from build123d import *

# Parameters (mm, degrees)
F2_R           = 14.99999
F4_D           = 5
F4_CBORE_D     = 8
F4_CBORE_DEPTH = 2


# Not quite as in the source:
# - a fillet or chamfer is up to 0.001 mm smaller than in the source, because OpenCascade refuses the exact size


with BuildPart() as f1:
    # F0 (on Front) → F1 (revolve)
    with BuildSketch(Plane.XZ):
        Polygon((36, -25), (0, -25), (0, -30), (43.5, -30), (43.5, -15), (36, -15), align=None)
    revolve(axis=Axis((0, 0, -27.5), (0, 0, 1)))

    # F2 (radius 15 in the source; OpenCascade refuses exactly that, so slightly less here)
    f2_edges = [f1.edges().sort_by_distance(p)[0] for p in [
        (-43.5, 0, -30),
    ]]
    fillet(f2_edges, radius=F2_R)

    # F4 (through all)
    with Locations(Plane(origin=(0, 0, -30), x_dir=(1, 0, 0), z_dir=(0, 0, -1))):
        with Locations((-12.9903810568, 7.5), (12.9903810568, 7.5), (0, -15)):
            CounterBoreHole(F4_D / 2, F4_CBORE_D / 2, F4_CBORE_DEPTH)


solid = f1.part
Geometry: final body of the model. Coordinates: model frame, mm. A direction names the side the tool comes from. Coordinates: 2 decimals unless noted, no trailing zeros. Write each loop counter-clockwise with the first axis right and the second up, starting at its lowest first coordinate (ties: lowest second). Pieces come first, ordered by that corner, then holes. Notation, with made-up numbers: (-39.5, -23) - (6.5, -23) arc R20 ccw to (6.5, -10) - close; hole circle Ø8 at (10, -11). An arc over 180 degrees is marked (long way). Return JSON: item names as keys, results as strings.
Item 1: Pull-direction query (Y, two-part tool) for faces 1 (the face through (0.54, 17.44, -26.48)), 2 (the face through (-16.3, 32.4, -15)), 3 (the face through (-4.686, 35.694, -20.07)); classes: +Y half, -Y half, draft (parallel to the pull), parting line (faces both ways), or undercut.
Completed:
{"face 1": "undercut", "face 2": "draft", "face 3": "undercut"}
Item 2: Pin query (flat end, axial travel): pin 1 Ø4 at (x, z) = (-21.5, -19) entering from -Y; pin 2 Ø10.5 at (x, y) = (-12.99, -7.5) entering from +Z; pin 3 Ø6.5 at (x, y) = (14, -8.5) entering from -Z; pin 4 Ø3 at (y, z) = (30, -27.5) entering from -X. Return the tip coordinate at first contact, or that it passes through.
Completed:
{"pin 1": "stops at y = -38.41", "pin 2": "stops at z = -25", "pin 3": "stops at z = -30", "pin 4": "stops at x = -25.01"}
Item 3: Section query D-D (z = -22.75). Output: boundary loops of the cut face in (x, y), and give its area (3 significant figures).
Completed:
{"outline": "circle Ø82.69 at (0, 0); hole circle Ø72 at (0, 0)", "area": "1,300 mm2"}
Item 4: Reachability of faces 4 (the face through (2, 13, -28)), 5 (the face through (11.8, -5.3, -26.5)), 6 (the face through (-1, 1, -25)) from +Z, -Z, +X, -X, +Y, -Y: full face, straight path, thin tool, end or side. Return the list, or none.
Completed:
{"face 4": "-Z", "face 5": "+Z, -Z", "face 6": "+Z"}
Item 5: Section query C-C (z = -16). Output: boundary loops of the cut face in (x, y).
Completed:
{"outline": "circle Ø86.93 at (0, 0); hole circle Ø72 at (0, 0)"}
Item 6: Line query: L1, parallel to Z at x = -4, y = 24.5; L2, parallel to Y at x = 23, z = -24.5; L3, parallel to X at y = 15, z = -17.75. Output: solid intervals per line, ascending.
Completed:
{"L1": "z = -30 to -25", "L2": "y = -32.86 to -27.69, 27.69 to 32.86", "L3": "x = -40.56 to -32.73, 32.73 to 40.56"}
